Input: part model. Units: mm. Frame: model coordinates. A direction names the side the tool comes from. Coordinates: 2 decimals unless noted, no trailing zeros. Write each loop counter-clockwise with the first axis right and the second up, starting at its lowest first coordinate (ties: lowest second). Pieces come first, ordered by that corner, then holes.
1) Section query A-A (y = 39.5). Output: boundary loops of the cut face in (x, z).
2) Draft query along Y for faces 5 (the flat face through (1, 1.5, 3)), 6 (the flat face through (1, 187, 10)), 7 (the flat face through (1, 94.5, 2)). Return one class per face: pulls with the +Y half, pulls with the -Y half, needs draft (parallel to the pull), parting line crosses it, or undercut.
3) Set-up query: faces 1 (the flat face through (1, 185, 0)), 2 (the flat face through (1, 5, 10)), 3 (the flat face through (1, 126.5, 2)), 4 (the flat face through (1, 0, 5)). Return all of +Z, -Z, +X, -X, +Y, -Y with unobstructed straight access to the full face (end or side cutting, diameter ignored); none if empty.
4) Pin query (flat end, axial travel): pin 1 Ø1.5 at (x, z) = (2, 11.5) entering from -Y; pin 2 Ø1.5 at (x, y) = (1, 187.5) entering from -Z; pin 3 Ø0.9 at (x, z) = (1.5, 3.5) entering from -Y. Return the tip coordinate at first contact, or that it passes through.
5) Line query: L1, parallel to Y at x = 1.75, z = 11; L2, parallel to Z at x = 1.7, y = 154. Output: solid intervals per line, ascending.
from build123d import *

# Parameters (mm, degrees)
F0_W     = 1.5
F0_H     = 5
F0_W_2   = 3
F0_H_2   = 2
F0_H_3   = 3
F1_DEPTH = 3


# Not quite as in the source:
# - a feature names something its author has since deleted; it is built from what else it names


with BuildPart() as f1:
    # F0 (on Right) → F1 (new body)
    with BuildSketch(Plane.YZ):
        Polygon((1.5, 5), (1.5, 0), (11.5, 0), (14.5, 0), (14.5, 5), (14.5, 10), (11.5, 10), (1.5, 10), align=None)
        with Locations((-0.75, 7.5)):
            Rectangle(F0_W, F0_H)
        with Locations((0.75, 7.5)):
            Rectangle(F0_W, F0_H)
        with Locations((13, -1)):
            Rectangle(F0_W_2, F0_H_2)
        with Locations((16, 7.5)):
            Rectangle(F0_W_2, F0_H)
        with Locations((19, -1)):
            Rectangle(F0_W_2, F0_H_2)
        Polygon((17.5, 5), (17.5, 0), (20.5, 0), (30.5, 0), (30.5, 5), (30.5, 10), (20.5, 10), (17.5, 10), align=None)
        with Locations((13, 11.5)):
            Rectangle(F0_W_2, F0_H_3)
        with Locations((16, 11.5)):
            Rectangle(F0_W_2, F0_H_3)
        with Locations((19, 11.5)):
            Rectangle(F0_W_2, F0_H_3)
        Polygon((33.5, 5), (33.5, 0), (43.5, 0), (46.5, 0), (46.5, 5), (46.5, 10), (33.5, 10), align=None)
        with Locations((32, 7.5)):
            Rectangle(F0_W_2, F0_H)
        with Locations((45, -1)):
            Rectangle(F0_W_2, F0_H_2)
        with Locations((48, 7.5)):
            Rectangle(F0_W_2, F0_H)
        with Locations((51, -1)):
            Rectangle(F0_W_2, F0_H_2)
        Polygon((49.5, 5), (49.5, 0), (52.5, 0), (62.5, 0), (62.5, 5), (62.5, 10), (49.5, 10), align=None)
        with Locations((64, 7.5)):
            Rectangle(F0_W_2, F0_H)
        Polygon((78.5, 10), (65.5, 10), (65.5, 5), (65.5, 0), (75.5, 0), (78.5, 0), (78.5, 5), align=None)
        with Locations((80, 7.5)):
            Rectangle(F0_W_2, F0_H)
        with Locations((77, -1)):
            Rectangle(F0_W_2, F0_H_2)
        Polygon((94.5, 10), (81.5, 10), (81.5, 5), (81.5, 0), (84.5, 0), (94.5, 0), (94.5, 5), align=None)
        with Locations((95.25, 7.5)):
            Rectangle(F0_W, F0_H)
        with Locations((83, -1)):
            Rectangle(F0_W_2, F0_H_2)
        with Locations((96.75, 7.5)):
            Rectangle(F0_W, F0_H)
        Polygon((110.5, 10), (97.5, 10), (97.5, 5), (97.5, 0), (107.5, 0), (110.5, 0), (110.5, 5), align=None)
        with Locations((112, 7.5)):
            Rectangle(F0_W_2, F0_H)
        Polygon((126.5, 10), (113.5, 10), (113.5, 5), (113.5, 0), (116.5, 0), (126.5, 0), (126.5, 5), align=None)
        with Locations((109, -1)):
            Rectangle(F0_W_2, F0_H_2)
        with Locations((128, 7.5)):
            Rectangle(F0_W_2, F0_H)
        with Locations((115, -1)):
            Rectangle(F0_W_2, F0_H_2)
        Polygon((142.5, 10), (129.5, 10), (129.5, 5), (129.5, 0), (139.5, 0), (142.5, 0), (142.5, 5), align=None)
        with Locations((144, 7.5)):
            Rectangle(F0_W_2, F0_H)
        Polygon((158.5, 10), (145.5, 10), (145.5, 5), (145.5, 0), (148.5, 0), (158.5, 0), (158.5, 5), align=None)
        with Locations((160, 7.5)):
            Rectangle(F0_W_2, F0_H)
        with Locations((141, -1)):
            Rectangle(F0_W_2, F0_H_2)
        with Locations((147, -1)):
            Rectangle(F0_W_2, F0_H_2)
        Polygon((171.5, 10), (161.5, 10), (161.5, 5), (161.5, 0), (171.5, 0), (174.5, 0), (174.5, 5), (174.5, 10), align=None)
        with Locations((173, 11.5)):
            Rectangle(F0_W_2, F0_H_3)
        with Locations((176, 11.5)):
            Rectangle(F0_W_2, F0_H_3)
        with Locations((176, 7.5)):
            Rectangle(F0_W_2, F0_H)
        with Locations((173, -1)):
            Rectangle(F0_W_2, F0_H_2)
        Polygon((180.5, 10), (177.5, 10), (177.5, 5), (177.5, 0), (180.5, 0), (190.5, 0), (190.5, 5), (190.5, 10), align=None)
        with Locations((179, 11.5)):
            Rectangle(F0_W_2, F0_H_3)
        with Locations((179, -1)):
            Rectangle(F0_W_2, F0_H_2)
        with Locations((191.25, 7.5)):
            Rectangle(F0_W, F0_H)
        with Locations((192.75, 7.5)):
            Rectangle(F0_W, F0_H)
    extrude(amount=F1_DEPTH)


solid = f1.part
Answer:
1. outline: (0, 0) - (3, 0) - (3, 10) - (0, 10) - close
2. face 5: pulls with the -Y half
2. face 6: needs draft
2. face 7: undercut
3. face 1: -Z, +X, -X, +Y
3. face 2: +Z, +X, -X, -Y
3. face 3: -Z, +X, -X
3. face 4: -Z, +X, -X, -Y
4. pin 1: stops at y = 11.5
4. pin 2: stops at z = 0
4. pin 3: stops at y = 1.5
5. L1: y = 11.5 to 20.5, 171.5 to 180.5
5. L2: z = 0 to 10
